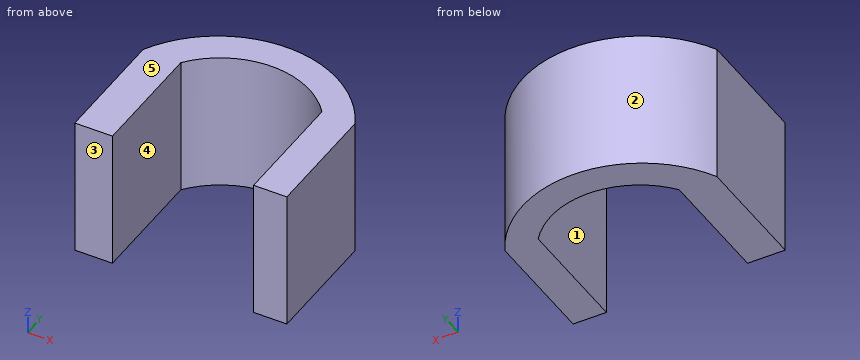
from build123d import *

# Parameters (mm, degrees)
F1_DEPTH = 50
F2_DEPTH = 50.001


with BuildPart() as f1:
    # F0 (on Top) → F1 (new body)
    with BuildSketch(Plane.XY):
        with BuildLine():
            Line((-33.415943, 42.985767), (-33.415943, 0))
            Line((-33.415943, 0), (-19.92406, 0))
            Line((-19.92406, 0), (-19.92406, 42.985767))
            ThreePointArc((-19.92406, 42.985767), (5.333999, 55.333899), (30.592058, 42.985767))
            Line((30.592058, 42.985767), (30.592058, 0))
            Line((30.592058, 0), (42.515114, 0))
            Line((42.515114, 0), (42.515114, 42.985767))
            ThreePointArc((42.515114, 42.985767), (4.549585, 66.042514), (-33.415943, 42.985767))
        make_face()
        with BuildLine():
            Line((-19.92406, 42.985767), (-19.92406, 0))
            Line((-19.92406, 0), (30.592058, 0))
            Line((30.592058, 0), (30.592058, 42.985767))
            ThreePointArc((30.592058, 42.985767), (5.333999, 55.333899), (-19.92406, 42.985767))
        make_face()
    extrude(amount=F1_DEPTH)

    # F0 (on Top) → F2 (cut, through all)
    with BuildSketch(Plane.XY):
        with BuildLine():
            Line((-19.92406, 42.985767), (-19.92406, 0))
            Line((-19.92406, 0), (30.592058, 0))
            Line((30.592058, 0), (30.592058, 42.985767))
            ThreePointArc((30.592058, 42.985767), (5.333999, 55.333899), (-19.92406, 42.985767))
        make_face()
    extrude(amount=F2_DEPTH, mode=Mode.SUBTRACT)


solid = f1.part
Geometry check sheet. Reference: the model listing, model coordinates, mm. Face numbers are marked on the shaded views. A direction names the side the tool comes from. Round coordinates to 2 decimals unless told otherwise and drop trailing zeros. Loops run counter-clockwise (first coordinate to the right, second up) from the corner with the lowest first, then second, coordinate; pieces in that order, holes last. Notation, with made-up numbers: (58, 10.25) -> (72, 10.25) arc R20 ccw to (72, 44.25) -> close; hole circle Ø1 at (-18.75, -13). An arc over 180 degrees is marked (long way). Answer as a JSON object with one key per item and string values. Group by question number.
Item 1: Cross-section at C-C, the plane x = -19. Record the cut outline in (y, z).
Item 2: Cross-section at B-B, the plane z = 15.5. Record the cut outline in (x, y).
Item 3: Thickness scan on line 1 along X through (y, z) = (38, 14.5); line 2 along Y through (x, z) = (-3, 35.5); line 3 along X through (y, z) = (50, 18.5). Record the ranges inside material, lowest first.
Item 4: Depth check by flat-ended pin: pin 1 Ø1.5 at (x, z) = (-22, 27) entering from +Y; pin 2 Ø10 at (x, y) = (-13, 17) entering from -Z; pin 3 Ø1.5 at (x, z) = (20.5, 8.5) entering from +Y; pin 4 Ø5 at (y, z) = (52, 22.5) entering from +X. Enter the tip coordinate at first touch or a pass-through.
Item 5: Release check for a two-part mould opening along X. For the marked faces 1, 2 and 3 record: pulls with the +X half, pulls with the -X half, needs draft (parallel to the pull), parting line crosses it, or undercut.
Item 6: Cross-section at A-A, the plane y = 31. Record the cut outline in (x, z).
Item 7: Cross-section at D-D, the plane y = 47. Record the cut outline in (x, z).
Item 8: Set-up check for the marked faces 4 and 5: record each of +Z, -Z, +X, -X, +Y, -Y from which the full face is reachable in a straight line by a thin tool's end or side.
Determined:
{
 "1": {"outline": "(44.12, 0) -> (58.98, 0) -> (58.98, 50) -> (44.12, 50) -> close"},
 "2": {"outline": "(-33.42, 0) -> (-19.92, 0) -> (-19.92, 42.99) arc R32.01 cw to (30.59, 42.99) -> (30.59, 0) -> (42.52, 0) -> (42.52, 42.99) arc R42.79 ccw to (-33.42, 42.99) -> close"},
 "3": {"line 1": "x = -33.42 to -19.92, 30.59 to 42.52", "line 2": "y = 54.23 to 65.37", "line 3": "x = -28.85 to -12.36, 23.03 to 37.95"},
 "4": {"pin 1": "stops at y = 57.39", "pin 2": "passes through", "pin 3": "stops at y = 63.25", "pin 4": "stops at x = 38.34"},
 "5": {"face 1": "undercut", "face 2": "parting line crosses it", "face 3": "needs draft"},
 "6": {"outline": "(-33.42, 0) -> (-19.92, 0) -> (-19.92, 50) -> (-33.42, 50) -> close; (30.59, 0) -> (42.52, 0) -> (42.52, 50) -> (30.59, 50) -> close"},
 "7": {"outline": "(-31.04, 0) -> (-16.21, 0) -> (-16.21, 50) -> (-31.04, 50) -> close; (26.88, 0) -> (40.14, 0) -> (40.14, 50) -> (26.88, 50) -> close"},
 "8": {"face 4": "+Z, -Z, -Y", "face 5": "+Z, +X, -X, +Y, -Y"}
}
